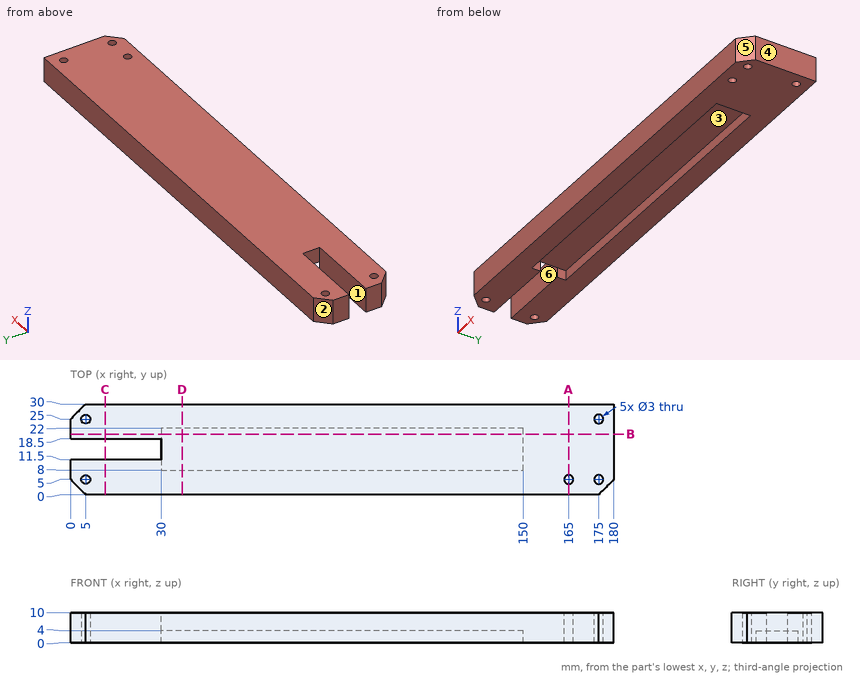
Geometry check sheet. Reference: drawing and pictorial views, mm from the part's lowest x, y, z. A direction names the side the tool comes from. Round coordinates to 2 decimals unless told otherwise and drop trailing zeros. Loops run counter-clockwise (first coordinate to the right, second up) from the corner with the lowest first, then second, coordinate; pieces in that order, holes last. Notation, with made-up numbers: (-10.5, 22.25) - (44.5, 22.25) arc R23 ccw to (44.5, 37.25) - close; hole circle Ø10 at (-16.75, -20.75). An arc over 180 degrees is marked (long way). Answer as CSV lines item,"result".
(1) Cross-section at C-C, the plane x = 11.5. Enter the section's corners in (y, z), and give its area (3 significant figures).
Output values:
outline,"(0, 0) - (11.5, 0) - (11.5, 10) - (0, 10) - close; (18.5, 0) - (30, 0) - (30, 10) - (18.5, 10) - close"
area,"230 mm²"
(2) Material ranges on line 1 along Y through (x, z) = (175, 4.5); line 2 along Y through (x, z) = (10, 0.75); line 3 along Y through (x, z) = (165, 7.5), recorded low to high.
Output values:
line 1,"y = 0 to 3.5, 6.5 to 23.5, 26.5 to 30"
line 2,"y = 0 to 11.5, 18.5 to 30"
line 3,"y = 0 to 3.5, 6.5 to 30"
(3) Release check for a two-part mould opening along Y. For the marked faces 3, 4, 5 and 6 record: released by +Y, released by -Y, zero draft, split by the parting line, or undercut.
Output values:
face 3,"undercut"
face 4,"zero draft"
face 5,"released by -Y"
face 6,"undercut"
(4) Cross-section at D-D, the plane x = 37. Enter the section's corners in (y, z).
Output values:
outline,"(0, 0) - (8, 0) - (8, 4) - (22, 4) - (22, 0) - (30, 0) - (30, 10) - (0, 10) - close"
(5) Cross-section at B-B, the plane y = 20. Enter the section's corners in (x, z).
Output values:
outline,"(0, 0) - (30, 0) - (30, 4) - (150, 4) - (150, 0) - (180, 0) - (180, 10) - (0, 10) - close"
(6) Depth check by flat-ended pin: pin 1 Ø2 at (y, z) = (15.5, 2.5) entering from -X; pin 2 Ø4 at (x, y) = (113.5, 12.5) entering from -Z. Enter the tip coordinate at first touch or a pass-through.
Output values:
pin 1,"stops at x = 150"
pin 2,"stops at z = 4"
(7) Cross-section at A-A, the plane x = 165. Enter the section's corners in (y, z).
Output values:
outline,"(0, 0) - (3.5, 0) - (3.5, 10) - (0, 10) - close; (6.5, 0) - (30, 0) - (30, 10) - (6.5, 10) - close"
(8) Set-up check for the marked faces 1 and 2: record each of +Z, -Z, +X, -X, +Y, -Y from which the full face is reachable in a straight line by a thin tool's end or side.
Output values:
face 1,"+Z, -Z, -X"
face 2,"+Z, -Z, -X, +Y"
